Source: three-view drawing plus pictorial views. Frame: mm from the lowest corner of the part. A direction names the side the tool comes from. Give positions to 0.01 mm unless a question says otherwise; leave off trailing zeros. Order: outer loops, then holes, each group sorted by start corner. A loop starts at its lowest first (then second) coordinate and runs counter-clockwise, first axis right, second up. Notation, with made-up numbers: (-28, 60) -> (24, 60) arc R12 cw to (24, 80) -> close; hole circle Ø3 at (22, -10). An arc over 180 degrees is marked (long way). Use a Markdown table: item, result. Add a question column.
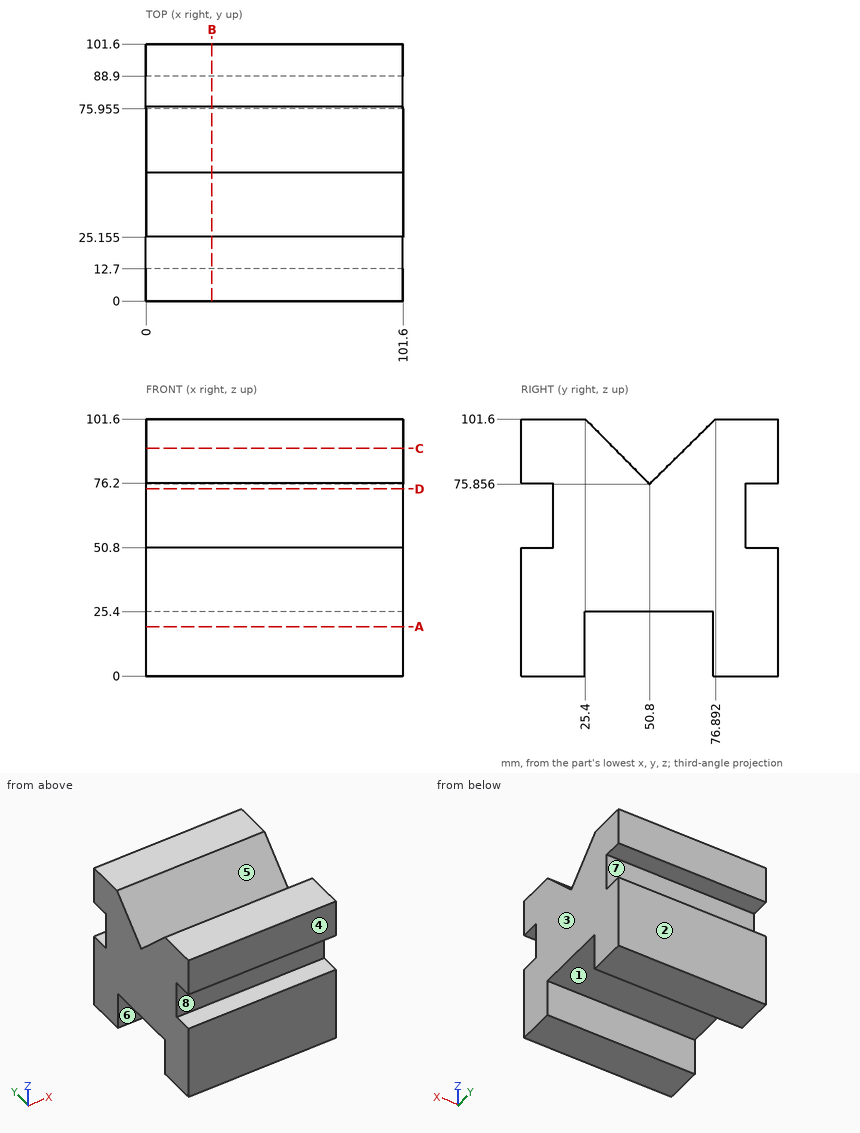
Q1. First-contact query: pin 1 (10 mm diameter, centred on x = 44.5, z = 68.5, fed in from -Y); pin 2 (12.5 mm diameter, centred on x = 69.5, z = 67.5, fed in from +Y); pin 3 (4 mm diameter, centred on x = 85, y = 59.5, fed in from -Z). Flat tips, straight axial feed; report the tip coordinate or a pass-through.
Q2. Section query B-B (x = 26). Return loops of the section in (y, z) (1 decimal).
Q3. Section query C-C (z = 90). Return loops of the section in (x, y) (1 decimal), plus the area to 3 significant figures.
Q4. Section query A-A (z = 19.5). Return loops of the section in (x, y) (1 decimal), plus the area to 3 significant figures.
Q5. Access query for the marked faces 5, 6, 7 and 8. Directions: +Z, -Z, +X, -X, +Y, -Y. A direction counts if a zero-diameter tool reaches every point of the face in a straight line with its end or side. Return the directions, or none.
Q6. Section query D-D (z = 74). Return loops of the section in (x, y), plus the area to 3 significant figures.
Q7. Ray query, line 1 (Y direction, x = 58, z = 9.5) (1 decimal); line 2 (Z direction, x = 22, y = 12); line 3 (Y direction, x = 93, z = 68). Return the intervals inside material, ascending.
Q8. Draft query along Y for the marked faces 1, 2, 3 and 4. Return one class per face: +Y half, -Y half, draft (parallel to the pull), parting line (faces both ways), or undercut.
Solution:
| question | item | result |
|---|---|---|
| 1 | pin 1 | stops at y = 12.7 |
| 1 | pin 2 | stops at y = 88.9 |
| 1 | pin 3 | stops at z = 25.4 |
| 2 | outline | (0, 0) -> (25.2, 0) -> (25.2, 25.4) -> (76, 25.4) -> (76, 0) -> (101.6, 0) -> (101.6, 50.8) -> (88.9, 50.8) -> (88.9, 76.2) -> (101.6, 76.2) -> (101.6, 101.6) -> (76.9, 101.6) -> (50.8, 75.9) -> (25.4, 101.6) -> (0, 101.6) -> (0, 76.2) -> (12.7, 76.2) -> (12.7, 50.8) -> (0, 50.8) -> close |
| 3 | outline | (0, 0) -> (101.6, 0) -> (101.6, 36.8) -> (0, 36.8) -> close; (0, 65.1) -> (101.6, 65.1) -> (101.6, 101.6) -> (0, 101.6) -> close |
| 3 | area | 7,450 mm² |
| 4 | outline | (0, 0) -> (101.6, 0) -> (101.6, 25.2) -> (0, 25.2) -> close; (0, 76) -> (101.6, 76) -> (101.6, 101.6) -> (0, 101.6) -> close |
| 4 | area | 5,160 mm² |
| 5 | face 5 | +Z, +X, -X |
| 5 | face 6 | -Z, +X, -X |
| 5 | face 7 | +X, -X, +Y |
| 5 | face 8 | +X, -X, -Y |
| 6 | outline | (0, 12.7) -> (101.6, 12.7) -> (101.6, 88.9) -> (0, 88.9) -> close |
| 6 | area | 7,740 mm² |
| 7 | line 1 | y = 0 to 25.2, 76 to 101.6 |
| 7 | line 2 | z = 0 to 50.8, 76.2 to 101.6 |
| 7 | line 3 | y = 12.7 to 88.9 |
| 8 | face 1 | undercut |
| 8 | face 2 | +Y half |
| 8 | face 3 | draft |
| 8 | face 4 | -Y half |
